Read the model definition and answer for the solid it produces. Units are mm, in the model's axes. A direction names the side the tool comes from. Round coordinates to 2 decimals unless told otherwise and drop trailing zeros. Order: outer loops, then holes, each group sorted by start corner. A loop starts at its lowest first (then second) coordinate and runs counter-clockwise, first axis right, second up. Notation, with made-up numbers: (-24.75, 52.25) -> (-17.75, 52.25) arc R21 ccw to (-17.75, 71.25) -> close; hole circle Ø6 at (-25, 7). An arc over 180 degrees is marked (long way). One line per item, written item: value. Start each with the question number.
1. The mould has two halves that part along Z. Classify faces 1 (the face through (96.995, 24.685, 1.201)), 2 (the face through (111.607, 24.615, 8.859)), 3 (the face through (87, 22.15, 0)), 4 (the face through (15.966, 2.465, -0.521)): released by +Z, released by -Z, zero draft, split by the parting line, or undercut.
2. Section A-A (x = 12) is taken. Give the vertices of the cut face in (y, z), then the cut area to 3 significant figures.
3. Section D-D (x = 87) is taken. Give the vertices of the cut face in (y, z), then the cut area to 3 significant figures.
4. Section B-B (y = 2.25) is taken. Give the vertices of the cut face in (x, z), then the cut area to 3 significant figures.
5. For faces 5 (the face through (112.81, 25, 0)), 6 (the face through (19, 5, 0)), determine the directions among +Z, -Z, +X, -X, +Y, -Y from which every point of the face is accessible in a straight line to the end or side of a thin tool.
6. Section C-C (y = 25.5) is taken. Give the vertices of the cut face in (x, z), then the cut area to 3 significant figures.
7. Flat-ended cylindrical pins translate along their axes: pin 1 Ø4 at (y, z) = (24.5, 6.5) entering from -X; pin 2 Ø10 at (x, z) = (21.5, 3.5) entering from +Y; pin 3 Ø6 at (y, z) = (10.5, 1.5) entering from -X. Find the tip coordinate at first contact, or state that the pin passes through.
8. Consider line 1 (Z direction, x = 100.81, y = 24.45); line 2 (Y direction, x = 17.5, z = 4.25); line 3 (Y direction, x = 92, z = -5). Determine where each line is inside the solid, lowest interval first.
from build123d import *

# Parameters (mm, degrees)
SKETCH1_R                    = 4
BASE_FLANGE1_DEPTH           = 5
EDGE_FLANGE1_STRIP_W         = 36
EDGE_FLANGE1_STRIP_H         = 5
EDGE_FLANGE1_STRIP_CUT_DEPTH = 20
EDGE_FLANGE1_DEPTH           = 20
EDGE_FLANGE2_STRIP_W         = 36
EDGE_FLANGE2_STRIP_H         = 5
EDGE_FLANGE2_STRIP_CUT_DEPTH = 20
EDGE_FLANGE2_DEPTH           = 20
SKETCH14_R                   = 4
CUT_EXTRUDE1_DEPTH           = 10
FILLET1_R                    = 4
FILLET3_R                    = 4
FILLET4_R                    = 10


# Sheet-metal steps are written as plain solids
with BuildPart() as part:
    # Sketch1 → Base-Flange1 (new body)
    with BuildSketch(Plane(origin=(0, 0, 0), x_dir=(1, 0, 0), z_dir=(0, 1, 0))):
        Polygon((4, 10), (0, 10), (0, 6), (0, -6), (0, -10), (4, -10), (47, -10), (47, 10), align=None)
        with Locations(Location((12, 0, 0), (0, 0, 270))):
            Circle(SKETCH1_R, mode=Mode.SUBTRACT)
    extrude(amount=BASE_FLANGE1_DEPTH)

    # Edge-Flange1 strip (across the edge) → Edge-Flange1 strip cut (cut)
    with BuildSketch(Plane(origin=(47, 5, 10), x_dir=(-1, 0, 0), z_dir=(0, 0, -1))):
        with Locations((-10, -2.5)):
            Rectangle(EDGE_FLANGE1_STRIP_W, EDGE_FLANGE1_STRIP_H)
    extrude(amount=EDGE_FLANGE1_STRIP_CUT_DEPTH, mode=Mode.SUBTRACT)

    # Edge-Flange1 section (across the edge) → Edge-Flange1 (add)
    with BuildSketch(Plane(origin=(47, 5, 10), x_dir=(-1, 0, 0), z_dir=(0, 0, -1))):
        with BuildLine():
            Line((-5, 8), (-5, 17.15))
            Line((-5, 17.15), (0, 17.15))
            Line((0, 17.15), (0, 8))
            ThreePointArc((0, 8), (2.343145751, 2.343145751), (8, 0))
            Line((8, 0), (8, -5))
            ThreePointArc((8, -5), (-1.192388155, -1.192388155), (-5, 8))
        make_face()
    extrude(amount=EDGE_FLANGE1_DEPTH)

    # Edge-Flange2 strip (across the edge) → Edge-Flange2 strip cut (cut)
    with BuildSketch(Plane(origin=(52, 22.15, -10), x_dir=(0, -1, 0), z_dir=(0, 0, 1))):
        with Locations((-10, -2.5)):
            Rectangle(EDGE_FLANGE2_STRIP_W, EDGE_FLANGE2_STRIP_H)
    extrude(amount=EDGE_FLANGE2_STRIP_CUT_DEPTH, mode=Mode.SUBTRACT)

    # Edge-Flange2 section (across the edge) → Edge-Flange2 (add)
    with BuildSketch(Plane(origin=(52, 22.15, -10), x_dir=(0, -1, 0), z_dir=(0, 0, 1))):
        with BuildLine():
            Line((-5, 8), (-5, 60.81))
            Line((-5, 60.81), (0, 60.81))
            Line((0, 60.81), (0, 8))
            ThreePointArc((0, 8), (2.343145751, 2.343145751), (8, 0))
            Line((8, 0), (8, -5))
            ThreePointArc((8, -5), (-1.192388155, -1.192388155), (-5, 8))
        make_face()
    extrude(amount=EDGE_FLANGE2_DEPTH)

    # Sketch14 → Cut-Extrude1 (cut)
    with BuildSketch(Plane(origin=(0, 27.15, 0), x_dir=(1, 0, 0), z_dir=(0, 1, 0))):
        with Locations(Location((100.81, 0, 0), (0, 0, 180))):
            Circle(SKETCH14_R)
    extrude(amount=-CUT_EXTRUDE1_DEPTH, mode=Mode.SUBTRACT)

    # Fillet1
    fillet1_edges = [part.edges().sort_by_distance(p)[0] for p in [
        (112.81, 24.65, -10),
        (112.81, 24.65, 10),
    ]]
    fillet(fillet1_edges, radius=FILLET1_R)

    # Fillet3
    fillet3_edges = [part.edges().sort_by_distance(p)[0] for p in [
        (0, 2.5, 10),
    ]]
    fillet(fillet3_edges, radius=FILLET3_R)

    # Fillet4
    fillet4_edges = [part.edges().sort_by_distance(p)[0] for p in [
        (0, 2.5, -10),
    ]]
    fillet(fillet4_edges, radius=FILLET4_R)


solid = part.part
Answer:
1. face 1: undercut
1. face 2: released by +Z
1. face 3: zero draft
1. face 4: undercut
2. outline: (0, -10) -> (5, -10) -> (5, -4) -> (0, -4) -> close; (0, 4) -> (5, 4) -> (5, 10) -> (0, 10) -> close
2. area: 60.0 mm^2
3. outline: (22.15, -10) -> (27.15, -10) -> (27.15, 10) -> (22.15, 10) -> close
3. area: 100 mm^2
4. outline: (0, 0) arc R10 ccw to (10, -10) -> (46.31, -10) -> (46.31, 10) -> (4, 10) arc R4 ccw to (0, 6) -> close; hole circle Ø8 at (12, 0)
4. area: 851 mm^2
5. face 5: +Z, -Z, +X, +Y, -Y
5. face 6: +Z, -Z, -X, +Y
6. outline: (53.66, -10) -> (108.81, -10) arc R4 ccw to (112.81, -6) -> (112.81, 6) arc R4 ccw to (108.81, 10) -> (53.66, 10) -> close; hole circle Ø8 at (100.81, 0)
6. area: 1,130 mm^2
7. pin 1: x = 50.04
7. pin 2: y = 5
7. pin 3: x = 44.81
8. line 1: -10 to -4, 4 to 10
8. line 2: 0 to 5
8. line 3: 22.15 to 27.15
